Source: three-view drawing plus pictorial views. Frame: mm from the lowest corner of the part. A direction names the side the tool comes from. Give positions to 0.01 mm unless a question says otherwise; leave off trailing zeros. Write item = value, one per line.
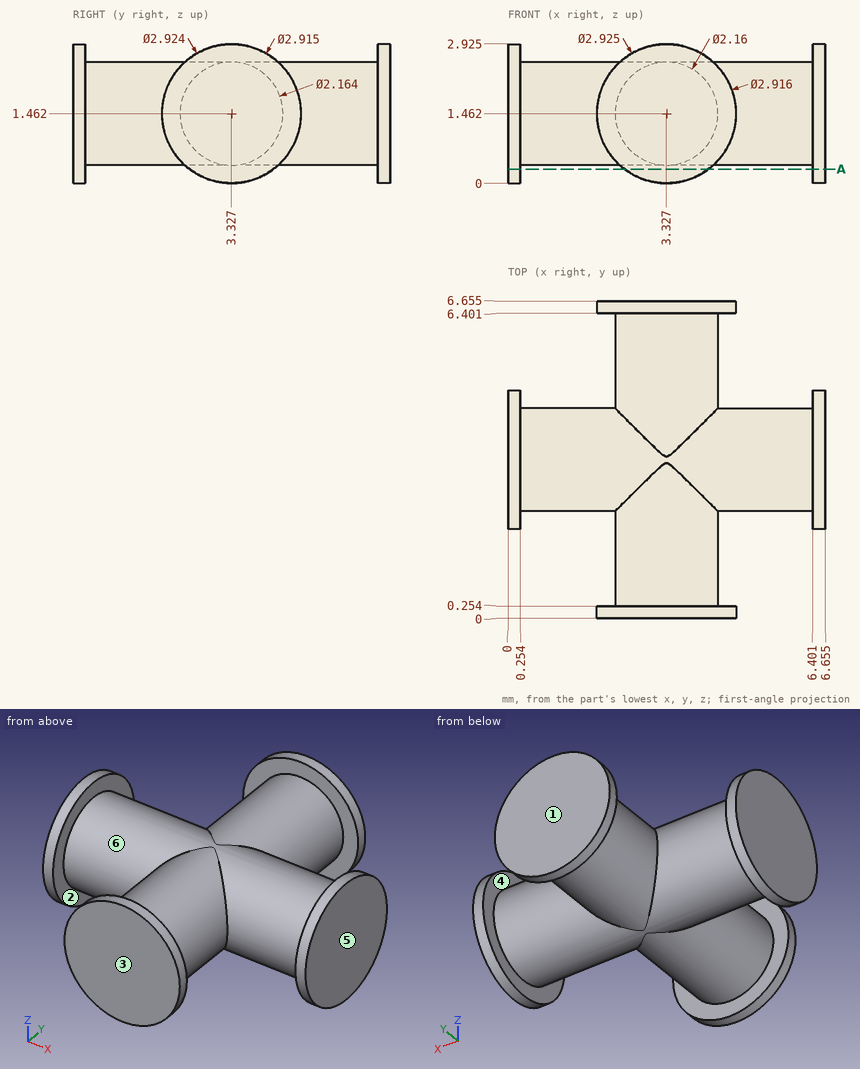
1) Line query: line 1 (X direction, y = 1.75, z = 2.3) (1 decimal); line 2 (Y direction, x = 6, z = 0.6) (1 decimal); line 3 (X direction, y = 5.5, z = 1.95) (1 decimal). Output: solid intervals per line, ascending. Write a range as from..to.
Check sheet entries:
line_1 = 2.6..4
line_2 = 2.7..4
line_3 = 2.4..4.3
2) Section query A-A (z = 0.3). Count the separate pieces of the cut face and the enclosed holes in it.
Check sheet entries:
separate_pieces = 4
enclosed_holes = 0
3) Mould query, pull axis X, two halves, no side actions, for the marked faces 3, 4, 5 and 6. Classes: +X half, -X half, draft (parallel to the pull), parting line (faces both ways), or undercut.
Check sheet entries:
face_3 = draft
face_4 = undercut
face_5 = +X half
face_6 = undercut
4) Reachability of the marked faces 1 and 2 from +Z, -Z, +X, -X, +Y, -Y: full face, straight path, thin tool, end or side. Return the list, or none.
Check sheet entries:
face_1 = +Z, -Z, +X, -X, +Y
face_2 = none
5) First-contact query: P1, Ø3, axis at x = 4, y = 4.5, coming from the +Z side (1 decimal). Flat tip, straight axial feed; report the tip coordinate or a pass-through.
Check sheet entries:
P1 = 2.5
